Part print with two shaded views. Sizes in mm from the minimum x, y, z corner. Round coordinates to 2 decimals unless told otherwise and drop trailing zeros. Write each loop counter-clockwise with the first axis right and the second up, starting at its lowest first coordinate (ties: lowest second). Pieces come first, ordered by that corner, then holes. Notation, with made-up numbers: (70, 37.5) -> (83, 37.5) arc R24 cw to (83, 61.5) -> close; hole circle Ø4 at (89.5, 12). An arc over 180 degrees is marked (long way). Answer as CSV lines item,"result".
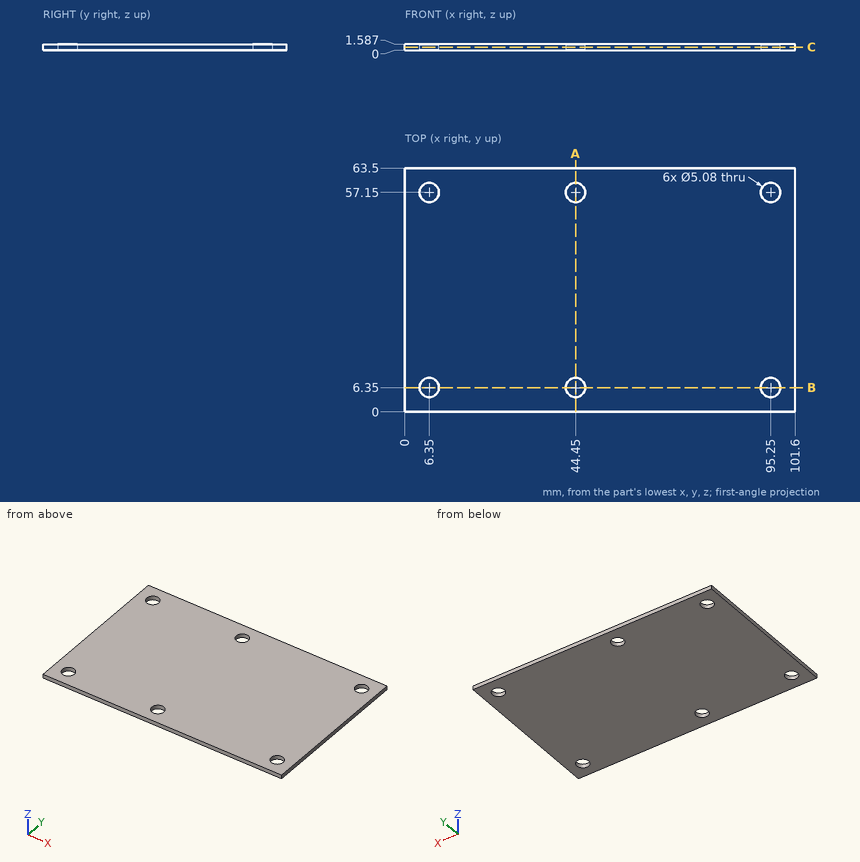
1. Drop a flat-ended pin along its axis: pin 1 Ø4.5 at (x, y) = (44.45, 6.35) entering from -Z. Give the stop position or say it passes through.
Results found:
pin 1,"passes through"
2. Cut at C-C, the plane z = 0.8. Write the cut outline in (x, y), then the cut area to 3 significant figures.
Results found:
outline,"(0, 0) -> (101.6, 0) -> (101.6, 63.5) -> (0, 63.5) -> close; hole circle Ø5.08 at (6.35, 6.35); hole circle Ø5.08 at (6.35, 57.15); hole circle Ø5.08 at (44.45, 6.35); hole circle Ø5.08 at (44.45, 57.15); hole circle Ø5.08 at (95.25, 6.35); hole circle Ø5.08 at (95.25, 57.15)"
area,"6,330 mm2"
3. Cut at B-B, the plane y = 6.35. Write the cut outline in (x, z).
Results found:
outline,"(0, 0) -> (3.81, 0) -> (3.81, 1.59) -> (0, 1.59) -> close; (8.89, 0) -> (41.91, 0) -> (41.91, 1.59) -> (8.89, 1.59) -> close; (46.99, 0) -> (92.71, 0) -> (92.71, 1.59) -> (46.99, 1.59) -> close; (97.79, 0) -> (101.6, 0) -> (101.6, 1.59) -> (97.79, 1.59) -> close"
4. Cut at A-A, the plane x = 44.45. Write the cut outline in (y, z).
Results found:
outline,"(0, 0) -> (3.81, 0) -> (3.81, 1.59) -> (0, 1.59) -> close; (8.89, 0) -> (54.61, 0) -> (54.61, 1.59) -> (8.89, 1.59) -> close; (59.69, 0) -> (63.5, 0) -> (63.5, 1.59) -> (59.69, 1.59) -> close"
5. Probe line 1 along Y through (x, z) = (44.45, 0.45); line 2 along Y through (x, z) = (97, 1.5); line 3 along X through (y, z) = (8, 0.75). List the from-to ranges inside material, lowest first.
Results found:
line 1,"y = 0 to 3.81, 8.89 to 54.61, 59.69 to 63.5"
line 2,"y = 0 to 4.51, 8.19 to 55.31, 58.99 to 63.5"
line 3,"x = 0 to 4.42, 8.28 to 42.52, 46.38 to 93.32, 97.18 to 101.6"
